Autodesk Inventor part; units mm, degrees
ref_plane "YZ Plane" through (0, 0, 0) normal (1, 0, 0) x (0, 1, 0)
ref_plane "XZ Plane" through (0, 0, 0) normal (0, 1, 0) x (-1, 0, 0)
ref_plane "XY Plane" through (0, 0, 0) normal (0, 0, 1) x (1, 0, 0)
sketch "Sketch1" plane through (0, 0, 0) normal (0, 1, 0) x (-1, 0, 0)
  line L0 (0, 0) -> (-37, 0)
  line L1 (-37, 0) -> (-37, 37)
  line L2 (-37, 37) -> (0, 37)
  line L3 (0, 37) -> (0, 0)
  circle A0 centre (-18.5, 18.5) radius 15.5
  point P0 (-18.5, 0)
  dimension "d0" = 37
  dimension "d1" = 37
  dimension "d2" = 18.5
  dimension "d3" = 18.5
  dimension "d4" = 31
extrude "Extrusion1" add sketch "Sketch1" against normal blind 20
sketch "Sketch3" plane through (0, 0, 37) normal (0, 0, 1) x (1, 0, 0)
  circle A0 centre (18.5, -10) radius 4.5
  line L0 (37, 0) -> (37, -20)
  point P0 (0, 0)
  dimension "d8" = 9
  dimension "d18" = 18.5
extrude "Extrusion2" cut sketch "Sketch3" against normal blind 5
sketch "Sketch4" plane through (37, 0, 0) normal (0, 0, -1) x (-1, 0, 0)
  circle A0 centre (18.5, -10) radius 4.5
  circle A1 centre (18.5, -10) radius 2.5
  point P0 (37, 0)
  dimension "d11" = 5
extrude "Extrusion3" cut sketch "Sketch4" against normal blind 5 contours A1
sketch "Sketch5" plane through (0, 0, 37) normal (0, 0, 1) x (1, 0, 0)
  line L0 (37, 0) -> (0, 0)
  line L1 (0, -20) -> (37, -20)
  line L2 (0, 0) -> (37, 0)
  line L3 (37, 0) -> (37, -20)
  line L4 (37, -20) -> (0, -20)
  line L5 (0, -20) -> (0, 0)
  line L6 (0, 0) -> (0, -20)
  line L7 (0, 0) -> (37, 0)
  line L8 (37, 0) -> (37, -20)
  line L9 (37, -20) -> (0, -20)
  line L10 (0, -20) -> (0, 0)
  circle A0 centre (18.5, -10) radius 4.5
  dimension "d19" = 18.5
extrude "Extrusion4" add sketch "Sketch5" along normal blind 2
sketch "Sketch6" plane through (0, 0, 39) normal (0, 0, 1) x (1, 0, 0)
  line L0 (0, 0) -> (0, -20)
  line L1 (0, -20) -> (37, -20)
  line L2 (0, 0) -> (37, 0)
  line L3 (37, 0) -> (37, -20)
  line L4 (37, -20) -> (0, -20)
  line L5 (0, -20) -> (0, 0)
  circle A0 centre (18.5, -10) radius 2.5
  dimension "d20" = 18.5
extrude "Extrusion5" add sketch "Sketch6" along normal blind 5
equation "\"d0\" = d1"
properties part number "welco mount v03"
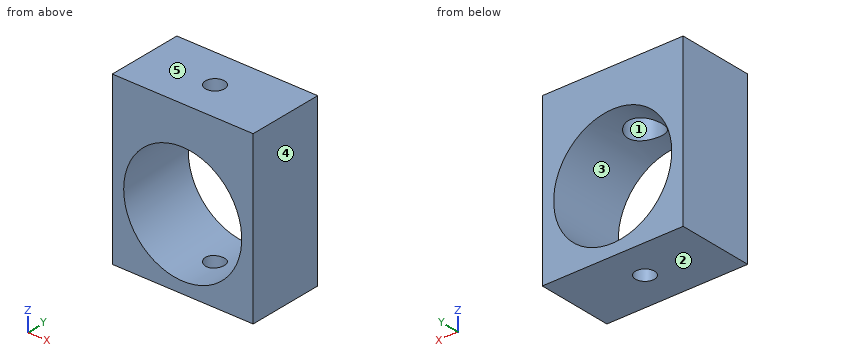
Could you check a few things on this model? Use its own coordinates, in mm. Face numbers are marked on the shaded views. A direction names the side the tool comes from. Coordinates: 2 decimals unless noted, no trailing zeros. Loops run counter-clockwise (first coordinate to the right, second up) from the corner with the lowest first, then second, coordinate; pieces in that order, holes last.
1. Imagine slicing it at D-D (y = -18). Please give me the cut outline in (x, z), and give its area (3 significant figures).
2. For P1, Ø6, axis at y = -5, z = 24.5, coming from the -X side, with a flat end and sliding along its axis, tell me the tip position at first contact or that it passes through.
3. Imagine slicing it at C-C (y = -10). Please give me the cut outline in (x, z), and give its area (3 significant figures).
4. I need wall thicknesses on L1, parallel to X at y = -10, z = 2.3; L2, parallel to Y at x = 18.5, z = 0.85; L3, parallel to Z at x = 18.5, y = -3. Which ranges of each line are inside material? Lowest first, please.
5. We'd pull the mould along Z, two halves only. Please class the marked faces 3, 4 and 5: released by +Z, released by -Z, zero draft, split by the parting line, or undercut.
6. Imagine slicing it at A-A (z = 18.5). Please give me the cut outline in (x, y), and give its area (3 significant figures).
7. Imagine slicing it at B-B (x = 18.5). Please give me the cut outline in (y, z), and give its area (3 significant figures).
8. For the marked faces 1 and 2, which set-ups out of +Z, -Z, +X, -X, +Y, -Y let a thin tool reach every point of the face, with its end or its side?
Computed values:
1. outline: (0, 0) - (37, 0) - (37, 44) - (0, 44) - close; hole circle Ø31 at (18.5, 18.5)
1. area: 873 mm2
2. P1: stops at x = 0
3. outline: (0, 0) - (16, 0) - (16, 3.2) arc R15.5 cw to (14, 33.33) - (14, 39) - (16, 39) - (16, 44) - (0, 44) - close; (21, 0) - (37, 0) - (37, 44) - (21, 44) - (21, 39) - (23, 39) - (23, 33.33) arc R15.5 cw to (21, 3.2) - close
3. area: 786 mm2
4. L1: x = 0 to 16, 21 to 37
4. L2: y = -20 to -12.5, -7.5 to 0
4. L3: z = 0 to 3, 34 to 44
5. face 3: undercut
5. face 4: zero draft
5. face 5: released by +Z
6. outline: (0, -20) - (3, -20) - (3, 0) - (0, 0) - close; (34, -20) - (37, -20) - (37, 0) - (34, 0) - close
6. area: 120 mm2
7. outline: (-20, 0) - (-12.5, 0) - (-12.5, 3) - (-20, 3) - close; (-20, 34) - (-14.5, 34) - (-14.5, 39) - (-12.5, 39) - (-12.5, 44) - (-20, 44) - close; (-7.5, 0) - (0, 0) - (0, 3) - (-7.5, 3) - close; (-7.5, 39) - (-5.5, 39) - (-5.5, 34) - (0, 34) - (0, 44) - (-7.5, 44) - close
7. area: 175 mm2
8. face 1: none
8. face 2: -Z, +X, -X, +Y, -Y
